```python
from build123d import *

# Parameters (mm, degrees)
F0_W     = 35.56
F0_H     = 76.2
F1_DEPTH = 38.1
F2_R     = 4.7625
F3_DEPTH = 0.254
F5_DEPTH = 127
F6_R     = 4.7625
F7_DEPTH = 0.254


with BuildPart() as f1:
    # F0 (on Top) → F1 (new body)
    with BuildSketch(Plane.XY):
        with BuildLine():
            Line((97.53417238, 58.7352159441), (-80.26582762, 58.7352159441))
            ThreePointArc((-80.26582762, 58.7352159441), (-89.2460837411, 55.0154720651), (-92.96582762, 46.0352159441))
            Line((-92.96582762, 46.0352159441), (-92.96582762, 33.3352159441))
            Line((-92.96582762, 33.3352159441), (-57.40582762, 33.3352159441))
            Line((-57.40582762, 33.3352159441), (74.67417238, 33.3352159441))
            Line((74.67417238, 33.3352159441), (110.23417238, 33.3352159441))
            Line((110.23417238, 33.3352159441), (110.23417238, 46.0352159441))
            ThreePointArc((110.23417238, 46.0352159441), (106.514428501, 55.0154720651), (97.53417238, 58.7352159441))
        make_face()
        with Locations((-75.18582762, -4.7647840559)):
            Rectangle(F0_W, F0_H)
        with Locations((92.45417238, -4.7647840559)):
            Rectangle(F0_W, F0_H)
    extrude(amount=F1_DEPTH)

    # F2 (on face) → F3 (join)
    with BuildSketch(Plane.XY.offset(38.1)):
        with Locations((-75.50332762, -19.0544008167)):
            Circle(F2_R)
        with Locations((92.77167238, -19.0544008167)):
            Circle(F2_R)
    extrude(amount=F3_DEPTH)

    # F4 (on face) → F5 (join)
    with BuildSketch(Plane(origin=(0, 58.7352159441, 0), x_dir=(-1, 0, 0), z_dir=(0, 1, 0))):
        with BuildLine():
            Line((-19.74667238, 19.05), (-8.63417238, 19.05))
            Line((-8.63417238, 19.05), (-8.63417238, 30.1625))
            ThreePointArc((-8.63417238, 30.1625), (-16.4918964859, 26.9077241059), (-19.74667238, 19.05))
        make_face()
        with BuildLine():
            Line((-8.63417238, 30.1625), (-8.63417238, 19.05))
            Line((-8.63417238, 19.05), (2.47832762, 19.05))
            ThreePointArc((2.47832762, 19.05), (-0.776448274, 26.9077241059), (-8.63417238, 30.1625))
        make_face()
        with BuildLine():
            Line((2.47832762, 19.05), (-8.63417238, 19.05))
            Line((-8.63417238, 19.05), (-8.63417238, 7.9375))
            ThreePointArc((-8.63417238, 7.9375), (-0.776448274, 11.1922758941), (2.47832762, 19.05))
        make_face()
        with BuildLine():
            Line((-8.63417238, 7.9375), (-8.63417238, 19.05))
            Line((-8.63417238, 19.05), (-19.74667238, 19.05))
            ThreePointArc((-19.74667238, 19.05), (-16.4918964859, 11.1922758941), (-8.63417238, 7.9375))
        make_face()
    extrude(amount=F5_DEPTH)

    # F6 (on face) → F7 (join)
    with BuildSketch(Plane(origin=(0, 0, 0), x_dir=(1, 0, 0), z_dir=(0, 0, -1))):
        with Locations((-75.50332762, 23.8147840559)):
            Circle(F6_R)
        with Locations((92.77167238, 23.8147840559)):
            Circle(F6_R)
    extrude(amount=F7_DEPTH)


solid = f1.part
```
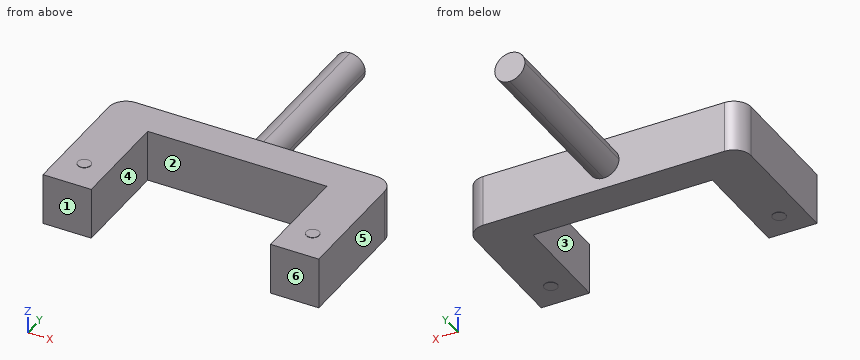
Part model, mm, in its own coordinate system. Face numbers are marked on the shaded views. A direction names the side the tool comes from. Round coordinates to 2 decimals unless told otherwise and drop trailing zeros. Loops run counter-clockwise (first coordinate to the right, second up) from the corner with the lowest first, then second, coordinate; pieces in that order, holes last. Notation, with made-up numbers: (69.25, 77) -> (122.25, 77) arc R21 ccw to (122.25, 82) -> close; hole circle Ø7 at (-7.75, 25.25). An arc over 180 degrees is marked (long way). Use a Markdown table: item, result.
1) Pull direction X, two halves, no side cores. Call the marked faces 3, 4, 5 and 6: pulls with the +X half, pulls with the -X half, needs draft (parallel to the pull), parting line crosses it, or undercut.
The answers:
| item | result |
|---|---|
| face 3 | undercut |
| face 4 | undercut |
| face 5 | pulls with the +X half |
| face 6 | needs draft |
2) Cut at B-B, the plane x = 17. List the corners of the cut face in (y, z), and give its area (3 significant figures).
The answers:
| item | result |
|---|---|
| outline | (33.34, 0) -> (58.74, 0) -> (58.74, 11.74) -> (185.74, 11.74) -> (185.74, 26.36) -> (58.74, 26.36) -> (58.74, 38.1) -> (33.34, 38.1) -> close |
| area | 2,830 mm2 |
3) Cut at A-A, the plane z = 3. List the corners of the cut face in (x, y).
The answers:
| item | result |
|---|---|
| outline | (-92.97, -42.86) -> (-57.41, -42.86) -> (-57.41, 33.34) -> (74.67, 33.34) -> (74.67, -42.86) -> (110.23, -42.86) -> (110.23, 46.04) arc R12.7 ccw to (97.53, 58.74) -> (-80.27, 58.74) arc R12.7 ccw to (-92.97, 46.04) -> close |
4) Probe line 1 (X direction, y = 13.5, z = 8.5); line 2 (Y direction, x = -30, z = 7); line 3 (Y direction, x = 83.5, z = 32.5). List the from-to ranges inside material, lowest first. Write a range as [from, to].
The answers:
| item | result |
|---|---|
| line 1 | x = [-92.97, -57.41], [74.67, 110.23] |
| line 2 | y = [33.34, 58.74] |
| line 3 | y = [-42.86, 58.74] |
5) Cut at D-D, the plane z = 16.5. List the corners of the cut face in (x, y), and give its area (3 significant figures).
The answers:
| item | result |
|---|---|
| outline | (-92.97, -42.86) -> (-57.41, -42.86) -> (-57.41, 33.34) -> (74.67, 33.34) -> (74.67, -42.86) -> (110.23, -42.86) -> (110.23, 46.04) arc R12.7 ccw to (97.53, 58.74) -> (19.45, 58.74) -> (19.45, 185.74) -> (-2.18, 185.74) -> (-2.18, 58.74) -> (-80.27, 58.74) arc R12.7 ccw to (-92.97, 46.04) -> close |
| area | 13,300 mm2 |
6) Drop flat-ended pins along their axis: pin 1 Ø12 at (y, z) = (154.5, 13) entering from +X; pin 2 Ø19 at (x, z) = (6, 12) entering from -Y; pin 3 Ø2 at (x, z) = (-32.5, 21) entering from +Y. Give the stop position or say it passes through.
The answers:
| item | result |
|---|---|
| pin 1 | stops at x = 19.75 |
| pin 2 | stops at y = 33.34 |
| pin 3 | stops at y = 58.74 |
7) Tool access for the marked faces 1 and 2: list every direction of +Z, -Z, +X, -X, +Y, -Y with a clear straight run to the whole face (end or side of a thin tool).
The answers:
| item | result |
|---|---|
| face 1 | +Z, -Z, +X, -X, -Y |
| face 2 | +Z, -Z, -Y |
